Check sheet for the modelled part. Datum: model origin and axes. Units: mm. Face numbers are marked on the shaded views. Coordinates: 2 decimals unless noted, no trailing zeros. Write each loop counter-clockwise with the first axis right and the second up, starting at its lowest first coordinate (ties: lowest second). Pieces come first, ordered by that corner, then holes. Notation, with made-up numbers: M 24,54 L 36,54 A27 ccw 36,76 Z; hole C 35.5,51 d11. An arc over 180 degrees is marked long. Answer as CSV lines item,"result". Start each with the question number.
Q1. Sectioned sample at D-D, the plane x = 90. Record the cut outline in (y, z), then the cut area to 3 significant figures.
Q2. Sectioned sample at C-C, the plane z = 3.5. Count the separate pieces of the cut face and the enclosed holes in it, then the cut area to 3 significant figures.
Q3. Thickness scan on line 1 along X through (y, z) = (-9, 0.5) (1 decimal); line 2 along Z through (x, y) = (0, -31); line 3 along Y through (x, z) = (44.5, -15). Record the ranges inside material, lowest first. Write a range as from..to.
Q4. Depth check by flat-ended pin: pin 1 Ø3 at (x, y) = (91, -21.5) entering from -Z; pin 2 Ø1.5 at (y, z) = (-36, 14) entering from -X; pin 3 Ø4 at (y, z) = (-37.5, -15.5) entering from +X. Enter the tip coordinate at first touch or a pass-through.
Q5. Sectioned sample at A-A, the plane x = 0. Record the cut outline in (y, z), then the cut area to 3 significant figures.
Q6. Mould release check, pull along Z, two halves, no side actions. Record for the marked faces 1, 2, 3 and 4: pulls with the +Z half, pulls with the -Z half, needs draft (parallel to the pull), parting line crosses it, or undercut.
Q7. Sectioned sample at B-B, the plane y = -16.5. Record the cut outline in (x, z), then the cut area to 3 significant figures.
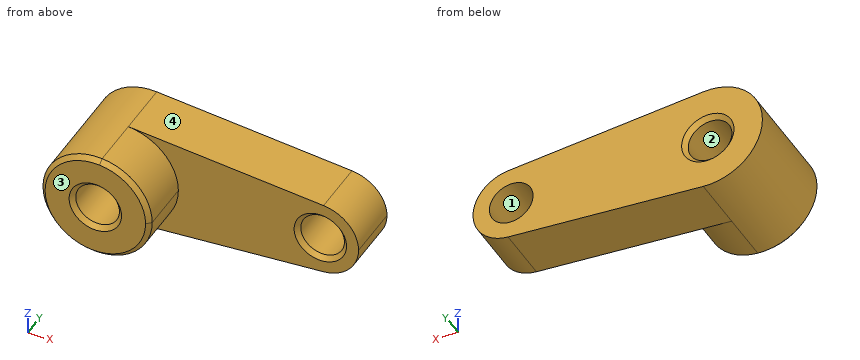
from build123d import *

# Parameters (mm, degrees)
F0_R     = 10
F1_DEPTH = 25
F2_DEPTH = 50
F3_SIZE  = 2


with BuildPart() as f1:
    # F0 (on Front) → F1 (new body)
    with BuildSketch(Plane.XZ):
        with BuildLine():
            ThreePointArc((2.083333, -24.913043), (18.399502, -16.92508), (25, 0))
            ThreePointArc((25, 0), (18.399502, 16.92508), (2.083333, 24.913043))
            ThreePointArc((2.083333, 24.913043), (-25, 0), (2.083333, -24.913043))
        make_face()
        Circle(F0_R, mode=Mode.SUBTRACT)
        with BuildLine():
            ThreePointArc((2.083333, 24.913043), (18.399502, 16.92508), (25, 0))
            ThreePointArc((25, 0), (18.399502, -16.92508), (2.083333, -24.913043))
            Line((2.083333, -24.913043), (91.458333, -17.43913))
            ThreePointArc((91.458333, -17.43913), (72.5, 0), (91.458333, 17.43913))
            Line((91.458333, 17.43913), (2.083333, 24.913043))
        make_face()
        with BuildLine():
            ThreePointArc((107.5, 0), (102.879651, 11.847556), (91.458333, 17.43913))
            ThreePointArc((91.458333, 17.43913), (72.5, 0), (91.458333, -17.43913))
            ThreePointArc((91.458333, -17.43913), (102.879651, -11.847556), (107.5, 0))
        make_face()
        with Locations((90, 0)):
            Circle(F0_R, mode=Mode.SUBTRACT)
    extrude(amount=F1_DEPTH)

    # F0 (on Front) → F2 (join)
    with BuildSketch(Plane.XZ):
        with BuildLine():
            ThreePointArc((2.083333, -24.913043), (18.399502, -16.92508), (25, 0))
            ThreePointArc((25, 0), (18.399502, 16.92508), (2.083333, 24.913043))
            ThreePointArc((2.083333, 24.913043), (-25, 0), (2.083333, -24.913043))
        make_face()
        Circle(F0_R, mode=Mode.SUBTRACT)
    extrude(amount=F2_DEPTH)

    # F3
    f3_edges = [f1.edges().sort_by_distance(p)[0] for p in [
        (-2.083333, -50, 24.913043),
        (-10, -50, 0),
        (-10, 0, 0),
        (10, -25, 0),
        (80, -25, 0),
    ]]
    chamfer(f3_edges, length=F3_SIZE)


solid = f1.part
Output:
1,outline,"M -25,-17.56 L 0,-17.56 L 0,-10 L -23,-10 L -25,-12 Z; M -25,12 L -23,10 L 0,10 L 0,17.56 L -25,17.56 Z"
1,area,"374 mm^2"
2,separate pieces,"3"
2,enclosed holes,"0"
2,area,"3,110 mm^2"
3,line 1,"x = -25..-10, 10..80, 100..107.5"
3,line 2,"z = -25..-10, 10..25"
3,line 3,"y = -25..0"
4,pin 1,"stops at z = -17.6"
4,pin 2,"stops at x = -21.2"
4,pin 3,"stops at x = 21.04"
5,outline,"M -50,-23 L -48,-25 L 0,-25 L 0,-12 L -2,-10 L -48,-10 L -50,-12 Z; M -50,12 L -48,10 L -2,10 L 0,12 L 0,25 L -48,25 L -50,23 Z"
5,area,"1,490 mm^2"
6,face 1,"undercut"
6,face 2,"undercut"
6,face 3,"needs draft"
6,face 4,"pulls with the +Z half"
7,outline,"M 2.08,-24.91 L 91.46,-17.44 A17.5 ccw 91.46,17.44 L 2.08,24.91 A25 ccw long Z; hole C 0,0 d20; hole C 90,0 d20"
7,area,"4,670 mm^2"
